Work out the finished part from the listing and answer in its coordinate system (mm). Face numbers are marked on the shaded views. A direction names the side the tool comes from. Coordinates: 2 decimals unless noted, no trailing zeros. Write each loop counter-clockwise with the first axis right and the second up, starting at its lowest first coordinate (ties: lowest second). Pieces come first, ordered by that corner, then holes. Notation, with made-up numbers: (12, 3) - (41, 3) arc R18 cw to (41, 22) - close; hole circle Ø3 at (35, 78). An arc over 180 degrees is marked (long way). Use a Markdown table: item, result. Add a question column.
(1) The part is cut by section D-D, the plane z = 5.75. Give the vertices of the cut face in (x, y), then the cut area to 3 significant figures.
(2) For a pull along X with two mould halves and no side action, classify the marked faces 5, 6, 7 and 8 as released by +X, released by -X, zero draft, split by the parting line, or undercut.
(3) Given pin 1 Ø3 at (y, z) = (6.5, 8.5) entering from -X; pin 2 Ø1.5 at (y, z) = (-6, 9) entering from +X; pin 3 Ø2 at (x, y) = (1, 2.5) entering from -Z; pin 4 Ø1.2 at (y, z) = (-6.5, 8.5) entering from -X, each flat-ended and moving along its own axis, determine where each tip first touches the part or whether it passes through.
(4) A tool of negligible diameter and unlimited length cuts with its end or side. For the marked faces 1, 2, 3 and 4, from which of +Z, -Z, +X, -X, +Y, -Y can it reach the whole face along a straight path? Write none if from no direction.
(5) The part is cut by section A-A, the plane x = 0. Give the vertices of the cut face in (y, z), then the cut area to 3 significant figures.
(6) Find the intervals of material crossed by line 1 (Y direction, x = -0.5, z = 8.5); line 2 (Y direction, x = -1.5, z = 10); line 3 (Z direction, x = 1, y = -6.5), in increasing order. Write a range as from..to.
(7) The part is cut by section C-C, the plane z = 8.5. Give the vertices of the cut face in (x, y).
Autodesk Inventor part; units mm, degrees
ref_plane "YZ Plane" through (0, 0, 0) normal (1, 0, 0) x (0, 1, 0)
ref_plane "XZ Plane" through (0, 0, 0) normal (0, 1, 0) x (-1, 0, 0)
ref_plane "XY Plane" through (0, 0, 0) normal (0, 0, 1) x (1, 0, 0)
sketch "Sketch1" plane through (0, 0, 0) normal (0, 0, 1) x (1, 0, 0)
  circle A0 centre (0, 0) radius 1.5
  line L0 (-3.25, 2.3318) -> (-3.25, -2.3318)
  arc A1 (-3.25, -2.3318) -> (3.25, -2.3318) centre (0, 0) ccw
  line L1 (3.25, -2.3318) -> (3.25, 2.3318)
  arc A2 (3.25, 2.3318) -> (-3.25, 2.3318) centre (0, 0) ccw
  line L2 (5, 4) -> (5, -4)
  line L3 (5, -4) -> (-5, -4)
  line L4 (-5, -4) -> (-5, 4)
  line L5 (-5, 4) -> (5, 4)
  line L6 (5, 4) -> (-5, -4) construction
  line L7 (5, -4) -> (-5, 4) construction
  dimension "d0" = 8
  dimension "d1" = 10
extrude "Extrusion1" add sketch "Sketch1" along normal blind 4 contours A0 | A2 L1 A1 L0 | L0 A1 L3 L4 L5 A2 | L5 L2 L3 A1 L1 A2
sketch "Sketch2" plane through (0, 0, 4) normal (0, 0, 1) x (1, 0, 0)
  line L0 (5, 4) -> (-5, 4)
  line L1 (-5, 4) -> (-5, -4)
  line L2 (-5, -4) -> (5, -4)
  line L3 (5, -4) -> (5, 4)
  circle A0 centre (0, 0) radius 1.5
  dimension "d4" = 3
extrude "Extrusion2" cut sketch "Sketch2" against normal blind 4 contours A0
sketch "Sketch3" plane through (0, 0, 0) normal (0, 0, -1) x (-1, 0, 0)
  circle A0 centre (0, 0) radius 1.5
  line L0 (-5, 4) -> (5, 4)
  line L1 (-5, -4) -> (-5, 4)
  line L2 (5, -4) -> (-5, -4)
  line L3 (5, 4) -> (5, -4)
  line L4 (-3.25, -2.3318) -> (-3.25, 2.3318)
  line L5 (3.25, 2.3318) -> (3.25, -2.3318)
  line L6 (-5, -4) -> (-3.25, -4)
  line L7 (-3.25, -4) -> (-3.25, 4)
  line L8 (-3.25, 4) -> (-5, 4)
  line L9 (-5, 4) -> (-5, -4)
  line L10 (5, 4) -> (5, -4)
  line L11 (5, -4) -> (3.25, -4)
  line L12 (3.25, -4) -> (3.25, 4)
  line L13 (3.25, 4) -> (5, 4)
  line L14 (5, 4) -> (5, -4)
  dimension "d7" = 1.75
  dimension "d8" = 8
  dimension "d9" = 1.75
  dimension "d10" = 8
extrude "Extrusion3" add sketch "Sketch3" along normal blind 4 contours L0 L7 L4 L2 L1 | L0 L3 L2 L12 L5
sketch "Sketch4" plane through (0, 0, 4) normal (0, 0, 1) x (1, 0, 0)
  circle A0 centre (0, 0) radius 1.5
  line L0 (5, 4) -> (-5, 4)
  line L1 (-5, 4) -> (-5, -4)
  line L2 (-5, -4) -> (5, -4)
  line L3 (5, -4) -> (5, 4)
  line L4 (5, -4) -> (-5, -4)
  line L5 (-5, -4) -> (-5, -9)
  line L6 (-5, -9) -> (5, -9)
  line L7 (5, -9) -> (5, -4)
  line L8 (5, -4) -> (5, 4)
  line L9 (5, 4) -> (-5, 4)
  line L10 (-5, 4) -> (-5, 9)
  line L11 (-5, 9) -> (5, 9)
  line L12 (5, 9) -> (5, 4)
  dimension "d13" = 10
  dimension "d14" = 5
  dimension "d15" = 10
  dimension "d16" = 5
extrude "Extrusion4" add sketch "Sketch4" along normal blind 8 contours L0 L10 L11 L12 | L7 L6 L5 L2
sketch "Sketch5" plane through (-3.25, -4, 0) normal (0, -1, 0) x (1, 0, 0)
  line L0 (0, 0) -> (6.5, 0)
  line L1 (6.5, 0) -> (6.5, -4)
  line L2 (8.25, -4) -> (6.5, -4)
  line L3 (8.25, -4) -> (8.25, 4)
  line L4 (-1.75, 4) -> (8.25, 4)
  line L5 (-1.75, -4) -> (-1.75, 4)
  line L6 (0, -4) -> (-1.75, -4)
  line L7 (0, 0) -> (0, -4)
  point P0 (3.25, 0)
extrude "Extrusion5" add sketch "Sketch5" along normal up to surface (5 mm away)
sketch "Sketch6" plane through (-3.25, 4, 0) normal (0, 1, 0) x (1, 0, 0)
  line L0 (6.5, 0) -> (0, 0)
  line L1 (0, 0) -> (0, 4)
  line L2 (-1.75, 4) -> (0, 4)
  line L3 (-1.75, 4) -> (-1.75, -4)
  line L4 (8.25, -4) -> (-1.75, -4)
  line L5 (8.25, -4) -> (8.25, 4)
  line L6 (6.5, 4) -> (8.25, 4)
  line L7 (6.5, 0) -> (6.5, 4)
  point P0 (3.25, 0)
extrude "Extrusion6" add sketch "Sketch6" along normal up to surface (5 mm away)
sketch "Sketch7" plane through (5, -9, -4) normal (1, 0, 0) x (0, 0, -1)
  line L0 (-8, 5) -> (-8, 13)
  line L1 (-8, 5) -> (-16, 5)
  line L2 (-16, 0) -> (-16, 5)
  line L3 (0, 0) -> (-16, 0)
  line L4 (0, 0) -> (0, 18)
  line L5 (0, 18) -> (-16, 18)
  line L6 (-16, 13) -> (-16, 18)
  line L7 (-8, 13) -> (-16, 13)
  line L8 (-8, 5) -> (-16, 5)
  line L9 (0, 0) -> (-16, 0)
  line L10 (-8, 5) -> (-16, 5)
  line L11 (-16, 5) -> (-16, 0)
  line L12 (-16, 0) -> (-8, 0)
  line L13 (-8, 0) -> (-8, 5)
  line L14 (-16, 18) -> (-16, 13)
  line L15 (-8, 13) -> (-16, 13)
  line L16 (-16, 13) -> (-16, 18)
  line L17 (-16, 18) -> (-8, 18)
  line L18 (-8, 18) -> (-8, 13)
  point P0 (-4, 9)
  point P1 (-8, 18)
  point P2 (-8, 0)
extrude "Extrusion7" cut sketch "Sketch7" against normal blind 3 contours L13 L3 L2 L1 | L7 L6 L5 L18
sketch "Sketch8" plane through (-5, -9, -4) normal (-1, 0, 0) x (0, 0, 1)
  line L0 (8, 18) -> (8, 13)
  line L1 (8, 5) -> (8, 0)
  line L2 (8, 13) -> (8, 5)
  line L3 (8, 13) -> (16, 13)
  line L4 (16, 18) -> (16, 13)
  line L5 (16, 18) -> (0, 18)
  line L6 (0, 18) -> (0, 0)
  line L7 (0, 0) -> (16, 0)
  line L8 (16, 5) -> (16, 0)
  line L9 (8, 5) -> (16, 5)
  point P0 (4, 9)
extrude "Extrusion8" cut sketch "Sketch8" against normal blind 3 contours L5 L4 L3 L0 | L9 L8 L7 L1
sketch "Sketch9" plane through (2, -9, -4) normal (1, 0, 0) x (0, 0, -1)
  line L0 (-8, 13) -> (-16, 13)
  line L1 (-8, 18) -> (-8, 13)
  line L2 (-16, 18) -> (-8, 18)
  line L3 (-16, 13) -> (-16, 18)
  line L4 (-16, 0) -> (-16, 5)
  line L5 (-8, 0) -> (-16, 0)
  line L6 (-8, 5) -> (-8, 0)
  line L7 (-16, 5) -> (-8, 5)
  line L8 (-16, 13) -> (-16, 18)
  line L9 (-16, 15.5) -> (-12.5, 15.5)
  circle A0 centre (-12.5, 15.5) radius 1
  line L10 (-16, 2.5) -> (-12.5, 2.5)
  circle A1 centre (-12.5, 2.5) radius 1
  point P0 (-4, 9)
  dimension "d27" = 3.5
  dimension "d28" = 2
  dimension "d29" = 3.5
  dimension "d30" = 2
extrude "Extrusion9" cut sketch "Sketch9" against normal blind 4 contours A0 | A1
chamfer "Chamfer1" distance 2 angle 45 2 edges at (5, 0, 4) (-5, 0, 4)
fillet "Fillet1" radius 1 4 edges at (2, 6.5, 4) (2, -6.5, 4) (-2, -6.5, 4) (-2, 6.5, 4)
properties part number "bbearing_holder_1"
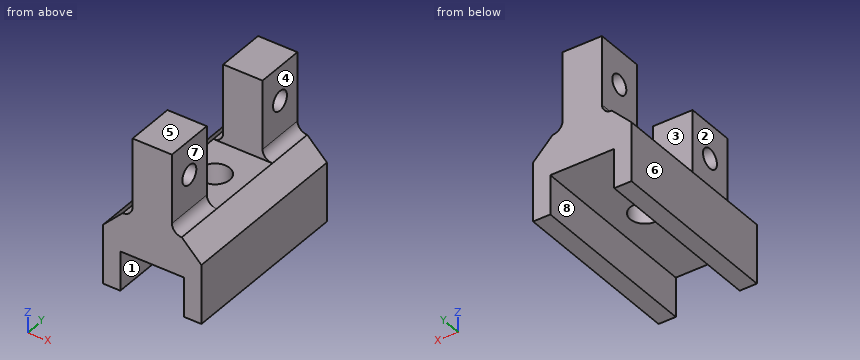
Model answer:
| question | item | result |
|---|---|---|
| 1 | outline | (-2, -9) - (2, -9) - (2, -4) - (-2, -4) - close; (-2, 4) - (2, 4) - (2, 9) - (-2, 9) - close |
| 1 | area | 40.0 mm^2 |
| 2 | face 5 | zero draft |
| 2 | face 6 | released by -X |
| 2 | face 7 | released by +X |
| 2 | face 8 | undercut |
| 3 | pin 1 | x = -2 |
| 3 | pin 2 | x = 2 |
| 3 | pin 3 | z = 0 |
| 3 | pin 4 | through |
| 4 | face 1 | -Z, +Y, -Y |
| 4 | face 2 | +Z, -X, +Y, -Y |
| 4 | face 3 | +Z, +X, -X |
| 4 | face 4 | +Z, +X, +Y, -Y |
| 5 | outline | (-9, 0) - (-1.5, 0) - (-1.5, 4) - (-4, 4) - (-4, 12) - (-9, 12) - close; (1.5, 0) - (9, 0) - (9, 12) - (4, 12) - (4, 4) - (1.5, 4) - close; hole circle Ø2 at (-6.5, 8.5); hole circle Ø2 at (6.5, 8.5) |
| 5 | area | 134 mm^2 |
| 6 | line 1 | -9..-7.5, -5.5..-4, 4..5.5, 7.5..9 |
| 6 | line 2 | -9..-4, 4..9 |
| 6 | line 3 | 0..7.5, 9.5..12 |
| 7 | outline | (-2, -9) - (2, -9) - (2, -7.5) - (-2, -7.5) - close; (-2, -5.5) - (2, -5.5) - (2, -4) - (-2, -4) - close; (-2, 4) - (2, 4) - (2, 5.5) - (-2, 5.5) - close; (-2, 7.5) - (2, 7.5) - (2, 9) - (-2, 9) - close |
